Geometry: final body of the model. Coordinates: model frame, mm. Give positions to 0.01 mm unless a question says otherwise; leave off trailing zeros. Write each loop counter-clockwise with the first axis right and the second up, starting at its lowest first coordinate (ties: lowest second). Pieces come first, ordered by that corner, then holes. Notation, with made-up numbers: M 8.5,87.5 L 64.5,87.5 A23 ccw 64.5,101.5 Z; hole C 11,64.5 d10. An arc over 180 degrees is marked long. Answer as a JSON object with one key per item and string values.
from build123d import *

# Parameters (mm, degrees)
SCHIZZO1_W                   = 25
SCHIZZO1_H                   = 25
ESTRUSIONE_ESTRUSIONE1_DEPTH = 1.5
TAGLIO_ESTRUSIONE1_DEPTH     = 18.741194999


with BuildPart() as part:
    # Schizzo1 → Estrusione-Estrusione1 (new body)
    with BuildSketch(Plane.XY):
        Rectangle(SCHIZZO1_W, SCHIZZO1_H)
    extrude(amount=ESTRUSIONE_ESTRUSIONE1_DEPTH)

    # Schizzo2 → Taglio-Estrusione1 (cut, through all)
    with BuildSketch(Plane.XY.offset(1.5)):
        with BuildLine():
            Line((-4, 0), (-4, -12.5))
            Line((-4, -12.5), (4, -12.5))
            Line((4, -12.5), (4, 0))
            ThreePointArc((4, 0), (0, 4), (-4, 0))
        make_face()
    extrude(amount=-TAGLIO_ESTRUSIONE1_DEPTH, mode=Mode.SUBTRACT)


solid = part.part
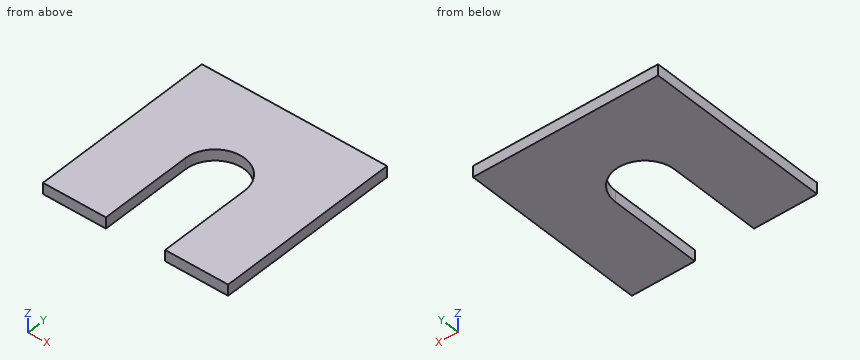
1) Cut plane D-D on x = 0. Return loops of the section in (y, z), and give its area (4 significant figures).
Geometry check:
{"outline": "M 4,0 L 12.5,0 L 12.5,1.5 L 4,1.5 Z", "area": "12.75 mm2"}
2) Cut plane C-C on y = 2.5. Return loops of the section in (x, z), and give its area (3 significant figures).
Geometry check:
{"outline": "M -12.5,0 L -3.12,0 L -3.12,1.5 L -12.5,1.5 Z; M 3.12,0 L 12.5,0 L 12.5,1.5 L 3.12,1.5 Z", "area": "28.1 mm2"}
3) Line query: line 1 (X direction, y = -11.5, z = 1.05); line 2 (Y direction, x = 0, z = 0.8); line 3 (X direction, y = 2, z = 1.35). Output: solid intervals per line, ascending. Write a range as from..to.
Geometry check:
{"line 1": "x = -12.5..-4, 4..12.5", "line 2": "y = 4..12.5", "line 3": "x = -12.5..-3.46, 3.46..12.5"}
4) Cut plane A-A on y = -0.5. Return loops of the section in (x, z), and give its area (3 significant figures).
Geometry check:
{"outline": "M -12.5,0 L -4,0 L -4,1.5 L -12.5,1.5 Z; M 4,0 L 12.5,0 L 12.5,1.5 L 4,1.5 Z", "area": "25.5 mm2"}
5) Cut plane B-B on z = 0.95. Return loops of the section in (x, y).
Geometry check:
{"outline": "M -12.5,-12.5 L -4,-12.5 L -4,0 A4 cw 4,0 L 4,-12.5 L 12.5,-12.5 L 12.5,12.5 L -12.5,12.5 Z"}
6) Contact query for a flat-ended pin moving along its axis: P1, Ø5, axis at x = -3, y = 9.5, coming from the -Z side. Output: stop coordinate, or through.
Geometry check:
{"P1": "stops at z = 0"}
